Autodesk Inventor part; units mm, degrees
ref_plane "YZ Plane" through (0, 0, 0) normal (1, 0, 0) x (0, 1, 0)
ref_plane "XZ Plane" through (0, 0, 0) normal (0, 1, 0) x (-1, 0, 0)
ref_plane "XY Plane" through (0, 0, 0) normal (0, 0, 1) x (1, 0, 0)
sketch "Boceto1" plane through (0, 0, 0) normal (0, 0, 1) x (1, 0, 0)
  line L0 (0, 0) -> (30, 0)
  line L1 (30, 0) -> (30, -30)
  line L2 (30, -30) -> (0, -30)
  line L3 (0, -30) -> (0, 0)
  dimension "d0" = 30
  dimension "d1" = 30
extrude "Extrusión1" add sketch "Boceto1" along normal blind 4
sketch "Boceto2" plane through (0, 0, 0) normal (0, 1, 0) x (1, 0, 0)
  line L0 (30, -4) -> (0, -4)
  line L1 (0, -4) -> (30, -4)
  line L2 (30, -4) -> (30, 26)
  line L3 (30, 26) -> (0, 26)
  line L4 (0, 26) -> (0, -4)
  point P0 (0, 0)
  dimension "d4" = 30
extrude "Extrusión2" add sketch "Boceto2" against normal blind 4
sketch "Boceto3" plane through (0, 0, 0) normal (0, 0, -1) x (-1, 0, 0)
  line L0 (0, -4) -> (-30, -4)
  line L1 (-30, -30) -> (-30, -4)
  line L2 (0, -30) -> (-30, -30)
  line L3 (0, -4) -> (0, -30)
  line L4 (0, -30) -> (-30, -30)
  line L5 (-15, -30) -> (-15, -4)
  line L6 (0, -4) -> (0, -30)
  line L7 (0, -17) -> (-30, -17)
  line L8 (-30, -17) -> (-22.5, -17)
  circle A0 centre (-22.5, -17) radius 3
  line L9 (0, -17) -> (-7.5, -17)
  circle A1 centre (-7.5, -17) radius 3
  point P0 (0, 0)
  dimension "d7" = 7.5
  dimension "d8" = 6
  dimension "d9" = 7.5
  dimension "d10" = 6
hole "Agujero1" at (22.5, -17, 0) at (7.5, -17, 0) direction (0, 0, 1) diameter 3.5 end through all countersink diameter 6 countersink angle 90
sketch "Boceto4" plane through (0, 0, 0) normal (0, 0, -1) x (-1, 0, 0)
  line L0 (0, -30) -> (-30, -30)
  line L1 (0, 0) -> (-3, 0)
  line L2 (-3, 0) -> (-3, -30)
  line L3 (-3, -30) -> (0, -30)
  line L4 (0, -30) -> (0, 0)
  line L5 (-30, -30) -> (-27, -30)
  line L6 (-27, -30) -> (-27, 0)
  line L7 (-27, 0) -> (-30, 0)
  line L8 (-30, 0) -> (-30, -30)
  dimension "d18" = 3
  dimension "d19" = 3
extrude "Extrusión3" add sketch "Boceto4" along normal up to surface (26 mm away)
sketch "Boceto5" plane through (30, -30, 4) normal (1, 0, 0) x (0, 0, -1)
  line L0 (30, 26) -> (4, 0)
  line L1 (30, 30) -> (0, 30)
  line L2 (0, 0) -> (0, 30)
  line L3 (30, 0) -> (0, 0)
  line L4 (30, 30) -> (30, 0)
  point P0 (4, 30)
extrude "Extrusión4" cut sketch "Boceto5" against normal through all contours L4 L3 L0
sketch "Boceto8" plane through (0, -4, 0) normal (0, -1, 0) x (1, 0, 0)
  line L0 (3, 0) -> (3, -26)
  line L1 (3, -26) -> (27, -26)
  line L2 (27, -26) -> (27, 0)
  line L3 (3, 0) -> (27, 0)
  line L4 (25.5, 0) -> (19.5, 0)
  line L5 (10.5, 0) -> (4.5, 0)
  line L6 (22.5, 0) -> (22.5, -26)
  line L7 (7.5, 0) -> (7.5, -26)
  line L8 (3, -26) -> (27, -26)
  line L9 (27, -26) -> (27, 0)
  line L10 (27, -13) -> (3, -13)
  circle A0 centre (22.5, -13) radius 1.75
  circle A1 centre (7.5, -13) radius 1.75
  point P0 (0, 0)
  dimension "d25" = 3.5
  dimension "d26" = 3.5
hole "Agujero2" at (22.5, -4, -13) at (7.5, -4, -13) direction (0, 1, 0) diameter 3.5 end through all countersink diameter 6 countersink angle 90
properties part number "Union"
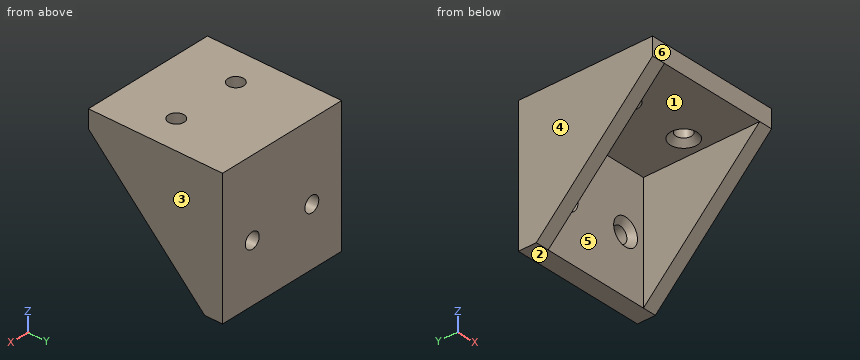
CAD build for the part. Positions are in the model's coordinates, mm. Face numbers are marked on the shaded views. A direction names the side the tool comes from. Give positions to 0.01 mm unless a question says otherwise; leave off trailing zeros. Order: outer loops, then holes, each group sorted by start corner. A loop starts at its lowest first (then second) coordinate and runs counter-clockwise, first axis right, second up.
(1) Saw through at C-C, the plane z = -13. Give the cut face in (x, y).
(2) Mould opens along X. For the marked faces 1, 2, 3 and 4 say: released by +X, released by -X, zero draft, split by the parting line, or undercut.
(3) Saw through at B-B, the plane y = -17. Give the cut face in (x, z), then the cut area to 3 significant figures.
(4) Saw through at D-D, the plane y = -23. Give the cut face in (x, z), then the cut area to 3 significant figures.
(5) Drill centre lines: L1, parallel to X at y = -1.05, z = -13; L2, parallel to X at y = -11.5, z = -17.5; L3, parallel to Y at x = 7.5, z = 3.2. Where is each one in solid material? Low to high.
(6) Flat gauge pins, fed straight in: pin 1 (7 mm diameter, centred on x = 10, y = -17, fed in from -Z); pin 2 (12 mm diameter, centred on x = 15.5, z = -13.5, fed in from -Y); pin 3 (5 mm diameter, centred on y = -23.5, z = -1.5, fed in from -X); pin 4 (5 mm diameter, centred on x = 27, y = -16, fed in from -Z). Where does each tip first touch, or does it go through?
(7) Saw through at A-A, the plane x = 22.5. Give the cut face in (y, z), then the cut area to 3 significant figures.
(8) Tool access for the marked faces 5 and 6: list every direction of +Z, -Z, +X, -X, +Y, -Y with a clear straight run to the whole face (end or side of a thin tool).
Results found:
1. outline: (0, -17) - (3, -17) - (3, -4) - (4.5, -4) - (5.75, -2.75) - (5.75, 0) - (0, 0) - close; (9.25, -2.75) - (10.5, -4) - (19.5, -4) - (20.75, -2.75) - (20.75, 0) - (9.25, 0) - close; (24.25, -2.75) - (25.5, -4) - (27, -4) - (27, -17) - (30, -17) - (30, 0) - (24.25, 0) - close
2. face 1: undercut
2. face 2: zero draft
2. face 3: released by +X
2. face 4: released by -X
3. outline: (0, -13) - (3, -13) - (3, 0) - (4.5, 0) - (5.75, 1.25) - (5.75, 4) - (0, 4) - close; (9.25, 1.25) - (10.5, 0) - (19.5, 0) - (20.75, 1.25) - (20.75, 4) - (9.25, 4) - close; (24.25, 1.25) - (25.5, 0) - (27, 0) - (27, -13) - (30, -13) - (30, 4) - (24.25, 4) - close
3. area: 167 mm2
4. outline: (0, -7) - (3, -7) - (3, 0) - (27, 0) - (27, -7) - (30, -7) - (30, 4) - (0, 4) - close
4. area: 162 mm2
5. L1: x = 0 to 5.75, 9.25 to 20.75, 24.25 to 30
5. L2: x = 0 to 3, 27 to 30
5. L3: y = -30 to -18.75, -15.25 to 0
6. pin 1: stops at z = 0
6. pin 2: stops at y = -4
6. pin 3: stops at x = 0
6. pin 4: stops at z = -16.5
7. outline: (-30, 0) - (-20, 0) - (-18.75, 1.25) - (-18.75, 4) - (-30, 4) - close; (-15.25, 1.25) - (-14, 0) - (-4, 0) - (-4, -10) - (-2.75, -11.25) - (0, -11.25) - (0, 4) - (-15.25, 4) - close; (-4, -26) - (0, -26) - (0, -14.75) - (-2.75, -14.75) - (-4, -16) - close
7. area: 193 mm2
8. face 5: -Z, -Y
8. face 6: +Z, -Z, +X, -X, -Y
